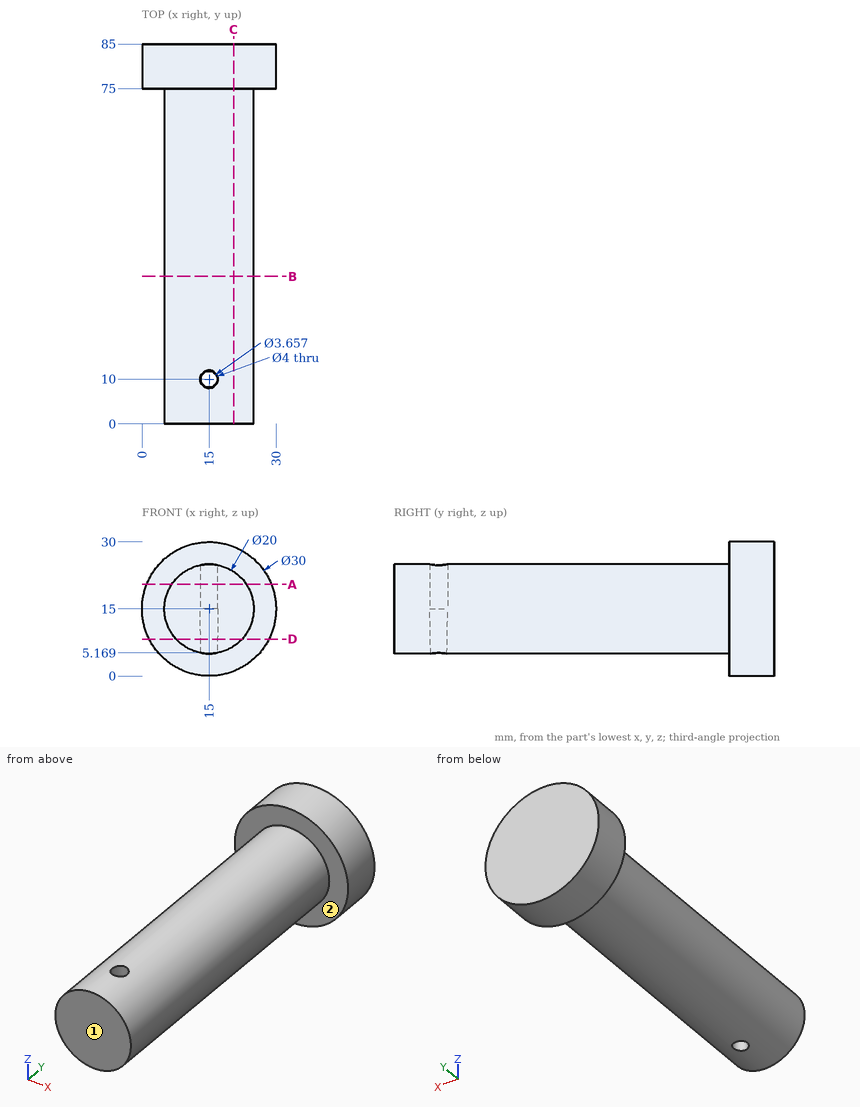
Design review of the part shown in the three views and the two pictorial views. Dimensions are in mm from the part's minimum x, y and z. A direction names the side the tool comes from. Coordinates: 2 decimals unless noted, no trailing zeros. Write each loop counter-clockwise with the first axis right and the second up, starting at its lowest first coordinate (ties: lowest second). Pieces come first, ordered by that corner, then holes.
1) To check wall thickness, follow probe 1 along Y at (x, z) = (15, 18); probe 2 along Y at (x, z) = (3.5, 18.25); probe 3 along X at (y, z) = (9.5, 13). State the ranges of each line that lie inside material, in increasing order.
2) We need section D-D on z = 8.25. State the section outline as (x, y) points (1 decimal), then the cut area to 3 significant figures.
3) Clearance check with flat-ended pins moving along their axes: pin 1 Ø5 at (x, y) = (15, 10) entering from +Z; pin 2 Ø2 at (y, z) = (66.5, 22) entering from +X; pin 3 Ø2 at (y, z) = (19.5, 14.5) entering from -X; pin 4 Ø5 at (x, z) = (25, 18.5) entering from -Y. State where each tip first meets the part, or that it passes through.
4) We need section B-B on y = 33. State the section outline as (x, z) points.
5) We need section C-C on x = 20.5. State the section outline as (y, z) points (1 decimal), then the cut area to 3 significant figures.
6) Machinability: for the marked faces 1 and 2, which of the approach directions +Z, -Z, +X, -X, +Y, -Y give a long, thin tool a straight path to every point of the face, cutting with its end or side? Answer none if there is none.
7) We need section A-A on z = 20.5. State the section outline as (x, y) points (1 decimal).
Answer list:
1. probe 1: y = 0 to 8, 12 to 85
1. probe 2: y = 75 to 85
1. probe 3: x = 5.2 to 13.1, 16.9 to 24.8
2. outline: (1.6, 75) - (7.6, 75) - (7.6, 0) - (22.4, 0) - (22.4, 75) - (28.4, 75) - (28.4, 85) - (1.6, 85) - close; hole circle Ø3.8 at (15, 10)
2. area: 1,360 mm2
3. pin 1: stops at z = 25
3. pin 2: stops at x = 23
3. pin 3: stops at x = 5
3. pin 4: stops at y = 0
4. outline: circle Ø20 at (15, 15)
5. outline: (0, 6.6) - (75, 6.6) - (75, 1) - (85, 1) - (85, 29) - (75, 29) - (75, 23.4) - (0, 23.4) - close
5. area: 1,530 mm2
6. face 1: +Z, -Z, +X, -X, -Y
6. face 2: -Y
7. outline: (1, 75) - (6.6, 75) - (6.6, 0) - (23.4, 0) - (23.4, 75) - (29, 75) - (29, 85) - (1, 85) - close; hole circle Ø4 at (15, 10)
